Verification items for the finished model (mm, model axes). Face numbers are marked on the shaded views. A direction names the side the tool comes from. Give positions to 0.01 mm unless a question says otherwise; leave off trailing zeros. Loops run counter-clockwise (first coordinate to the right, second up) from the corner with the lowest first, then second, coordinate; pieces in that order, holes last. Notation, with made-up numbers: (68, 27.5) - (114, 27.5) arc R7 cw to (114, 40.5) - close; hole circle Ø1 at (19.5, -39). An arc over 180 degrees is marked (long way). Use one line per item in the form item = value.
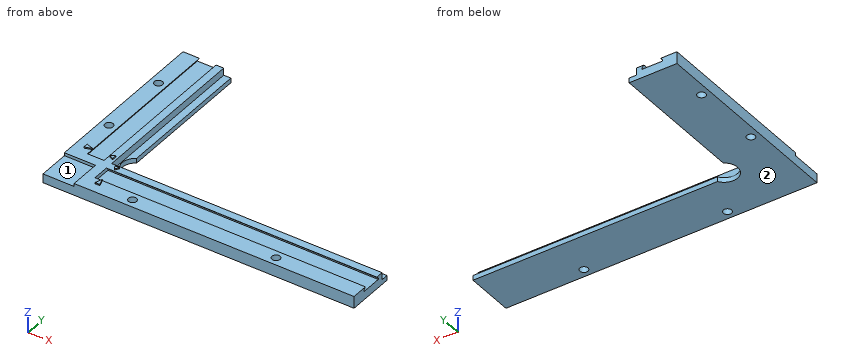
```python
from build123d import *

# Parameters (mm, degrees)
PAD_DEPTH       = 5
POCKET_DEPTH    = 113
SKETCH002_W     = 4
SKETCH002_H     = 4
POCKET001_DEPTH = 113
SKETCH003_W     = 3.38924
SKETCH003_H     = 4
POCKET002_DEPTH = 68
POCKET003_DEPTH = 68
SKETCH005_W     = 14
SKETCH005_H     = 14
POCKET004_DEPTH = 1.25
PAD001_DEPTH    = 0.5
SKETCH007_R     = 5.673714
POCKET005_DEPTH = 5
SKETCH008_R     = 1.7
POCKET006_DEPTH = 5.501


with BuildPart() as part:
    # Sketch → Pad (new body)
    with BuildSketch(Plane.XY):
        Polygon((0, 0), (0, 85), (20, 85), (20, 20), (130, 20), (130, 0), align=None)
    extrude(amount=PAD_DEPTH)

    # Sketch001 → Pocket (cut)
    with BuildSketch(Plane.YZ.offset(130)):
        Polygon((6, 3.5), (6, 4.1), (8.557521, 6.657521), (12.142479, 6.657521), (14.7, 4.1), (14.7, 3.5), align=None)
    extrude(amount=-POCKET_DEPTH, mode=Mode.SUBTRACT)

    # Sketch002 → Pocket001 (cut)
    with BuildSketch(Plane.YZ.offset(130)):
        with Locations((19, 4)):
            Rectangle(SKETCH002_W, SKETCH002_H)
    extrude(amount=-POCKET001_DEPTH, mode=Mode.SUBTRACT)

    # Sketch003 → Pocket002 (cut)
    with BuildSketch(Plane(origin=(0, 85, 0), x_dir=(-1, 0, 0), z_dir=(0, 1, 0))):
        with Locations((-18.69462, 4)):
            Rectangle(SKETCH003_W, SKETCH003_H)
    extrude(amount=-POCKET002_DEPTH, mode=Mode.SUBTRACT)

    # Sketch004 → Pocket003 (cut)
    with BuildSketch(Plane(origin=(0, 85, 0), x_dir=(-1, 0, 0), z_dir=(0, 1, 0))):
        Polygon((-14.7, 3.5), (-14.7, 4.1), (-13.019806, 5.780194), (-7.680194, 5.780194), (-6, 4.1), (-6, 3.5), align=None)
    extrude(amount=-POCKET003_DEPTH, mode=Mode.SUBTRACT)

    # Sketch005 → Pocket004 (cut)
    with BuildSketch(Plane.XY.offset(5)):
        with Locations((6, 6)):
            Rectangle(SKETCH005_W, SKETCH005_H)
    extrude(amount=-POCKET004_DEPTH, mode=Mode.SUBTRACT)

    # Sketch006 → Pad001 (new body)
    with BuildSketch(Plane.XY.offset(5)):
        Polygon((20, 7), (19, 4), (21, 4), align=None)
        Polygon((20, 14.44055), (19, 16), (21, 16), align=None)
        Polygon((14, 20), (16, 19), (16, 21), align=None)
        Polygon((7, 20), (4, 21), (4, 19), align=None)
    extrude(amount=PAD001_DEPTH)

    # Sketch007 → Pocket005 (cut)
    with BuildSketch(Plane(origin=(0, 0, 0), x_dir=(1, 0, 0), z_dir=(0, 0, -1))):
        with Locations((23, -23)):
            Circle(SKETCH007_R)
    extrude(amount=-POCKET005_DEPTH, mode=Mode.SUBTRACT)

    # Sketch008 → Pocket006 (cut, through all)
    with BuildSketch(Plane(origin=(0, 0, 0), x_dir=(1, 0, 0), z_dir=(0, 0, -1))):
        with Locations((35, -3.5)):
            Circle(SKETCH008_R)
        with Locations((95, -3.5)):
            Circle(SKETCH008_R)
        with Locations((3.5, -35)):
            Circle(SKETCH008_R)
        with Locations((3.5, -65)):
            Circle(SKETCH008_R)
    extrude(amount=-POCKET006_DEPTH, mode=Mode.SUBTRACT)


solid = part.part
```
1. Section check D-D, the plane y = 69.5. Record the cut outline in (x, z), then the cut area to 3 significant figures.
Result set:
outline = (0, 0) - (20, 0) - (20, 2) - (17, 2) - (17, 5) - (13.8, 5) - (14.7, 4.1) - (14.7, 3.5) - (6, 3.5) - (6, 4.1) - (6.9, 5) - (0, 5) - close
area = 78.8 mm²
2. Section check B-B, the plane x = 35. Record the cut outline in (y, z).
Result set:
outline = (0, 0) - (1.8, 0) - (1.8, 5) - (0, 5) - close; (5.2, 0) - (20, 0) - (20, 2) - (17, 2) - (17, 5) - (13.8, 5) - (14.7, 4.1) - (14.7, 3.5) - (6, 3.5) - (6, 4.1) - (6.9, 5) - (5.2, 5) - close
3. Depth check by flat-ended pin: pin 1 Ø7 at (x, y) = (9, 39) entering from +Z; pin 2 Ø2 at (x, z) = (51, 0.5) entering from +Y; pin 3 Ø1.5 at (x, z) = (83, 3) entering from +Y; pin 4 Ø2 at (x, y) = (3.5, 35) entering from +Z. Enter the tip coordinate at first touch or a pass-through.
Result set:
pin_1 = 5
pin_2 = 20
pin_3 = 17
pin_4 = through
4. Section check A-A, the plane z = 0.85. Record the cut outline in (x, y), then the cut area to 3 significant figures.
Result set:
outline = (0, 0) - (130, 0) - (130, 20) - (27.82, 20) arc R5.67 cw (long way) to (20, 27.82) - (20, 85) - (0, 85) - close; hole circle Ø3.4 at (3.5, 35); hole circle Ø3.4 at (3.5, 65); hole circle Ø3.4 at (35, 3.5); hole circle Ø3.4 at (95, 3.5)
area = 3,830 mm²
5. Tool access check on the marked faces 1 and 2. Record the directions out of +Z, -Z, +X, -X, +Y, -Y that give a thin tool (end or side, any length) a straight path to the whole face; none if there is none.
Result set:
face_1 = +Z, -X, -Y
face_2 = -Z, +X, -X, +Y, -Y
6. Scan lines: probe 1 along X at (y, z) = (3.5, 1.35); probe 2 along Y at (x, z) = (95, 3.8); probe 3 along X at (y, z) = (65, 1.55). Record each from-to range of solid material in increasing order.
Result set:
probe_1 = 0 to 33.3, 36.7 to 93.3, 96.7 to 130
probe_2 = 0 to 1.8, 5.2 to 6, 14.7 to 17
probe_3 = 0 to 1.8, 5.2 to 20
